```python
from build123d import *

# Parameters (mm, degrees)
ESQUISSE1_W             = 43
ESQUISSE1_H             = 43
BOSS_EXTRU_1_DEPTH      = 40
ESQUISSE2_W             = 48
ESQUISSE2_H             = 48
BOSS_EXTRU_2_DEPTH      = 1.5
ENL_V_MAT_EXTRU_3_REACH = 50
ESQUISSE5_W             = 8
ESQUISSE5_H             = 5
ENL_V_MAT_EXTRU_4_REACH = 43.5
ESQUISSE6_W             = 54.781223227
ESQUISSE6_H             = 3.078773465


with BuildPart() as part:
    # Esquisse1 → Boss.-Extru.1 (new body)
    with BuildSketch(Plane.XY):
        Polygon((-2.5, 43), (-2.5, -2.5), (0, -2.5), (45.5, -2.5), (45.5, 43), (45.5, 45.5), (-2.5, 45.5), align=None)
        with Locations((21.5, 21.5)):
            Rectangle(ESQUISSE1_W, ESQUISSE1_H, mode=Mode.SUBTRACT)
    extrude(amount=BOSS_EXTRU_1_DEPTH)

    # Esquisse2 → Boss.-Extru.2 (add)
    with BuildSketch(Plane.XY):
        with Locations((21.5, 21.5)):
            Rectangle(ESQUISSE2_W, ESQUISSE2_H)
    extrude(amount=-BOSS_EXTRU_2_DEPTH)

    # Esquisse5 → Enlèv. mat.-Extru.3 (cut, up to next)
    with BuildSketch(Plane(origin=(0, 45.5, 0), x_dir=(1, 0, 0), z_dir=(0, 1, 0)), mode=Mode.PRIVATE) as enl_v_mat_extru_3_sk1:
        with Locations((21.5, -6.3)):
            Rectangle(ESQUISSE5_W, ESQUISSE5_H)
    enl_v_mat_extru_3_tool1 = extrude(enl_v_mat_extru_3_sk1.sketch, amount=-ENL_V_MAT_EXTRU_3_REACH, mode=Mode.PRIVATE) & part.part
    add(enl_v_mat_extru_3_tool1.solids().sort_by_distance((21.5, 45.5, 6.3))[0], mode=Mode.SUBTRACT)

    # Esquisse6 → Enlèv. mat.-Extru.4 (cut, up to next)
    with BuildSketch(Plane.XY.offset(40), mode=Mode.PRIVATE) as enl_v_mat_extru_4_sk1:
        with Locations((23.162986277, -1.539386733)):
            Rectangle(ESQUISSE6_W, ESQUISSE6_H)
    enl_v_mat_extru_4_tool1 = extrude(enl_v_mat_extru_4_sk1.sketch, amount=-ENL_V_MAT_EXTRU_4_REACH, mode=Mode.PRIVATE) & part.part
    add(enl_v_mat_extru_4_tool1.solids().sort_by_distance((23.162986, -1.539387, 40))[0], mode=Mode.SUBTRACT)


solid = part.part
```
Verification items for the finished model (mm, model axes). A direction names the side the tool comes from. Give positions to 0.01 mm unless a question says otherwise; leave off trailing zeros. Loops run counter-clockwise (first coordinate to the right, second up) from the corner with the lowest first, then second, coordinate; pieces in that order, holes last. Notation, with made-up numbers: M 26,59.25 L 50,59.25 A25 ccw 50,86.25 Z; hole C 29,34.25 d9. An arc over 180 degrees is marked long. One line per question, with ' | ' between items.
Item 1: Depth check by flat-ended pin: P1, Ø20, axis at x = 15.5, z = 20.5, coming from the -Y side; P2, Ø13, axis at x = 22.5, y = 18.5, coming from the +Z side. Enter the tip coordinate at first touch or a pass-through.
Completed:
P1: stops at y = 43 | P2: stops at z = 0
Item 2: Tool access check on faces 1 (the face through (17.5, 44, 6)), 2 (the face through (45.5, 22, 20)), 3 (the face through (0, 21, 20)). Record the directions out of +Z, -Z, +X, -X, +Y, -Y that give a thin tool (end or side, any length) a straight path to the whole face; none if there is none.
Completed:
face 1: +Y, -Y | face 2: +Z, -Z, +X, +Y, -Y | face 3: +Z, -Y
Item 3: Thickness scan on line 1 (X direction, y = 29, z = 8); line 2 (Z direction, x = 18, y = 13); line 3 (Y direction, x = 6, z = 20). Record the ranges inside material, lowest first. Write a range as [from, to].
Completed:
line 1: x = [-2.5, 0], [43, 45.5] | line 2: z = [-1.5, 0] | line 3: y = [43, 45.5]
Item 4: Section check C-C, the plane y = 20.5. Record the cut outline in (x, z), plus the area to 3 significant figures.
Completed:
outline: M -2.5,-1.5 L 45.5,-1.5 L 45.5,40 L 43,40 L 43,0 L 0,0 L 0,40 L -2.5,40 Z | area: 272 mm^2
Item 5: Section check B-B, the plane x = 22.5. Record the cut outline in (y, z).
Completed:
outline: M 0,-1.5 L 45.5,-1.5 L 45.5,3.8 L 43,3.8 L 43,0 L 0,0 Z; M 43,8.8 L 45.5,8.8 L 45.5,40 L 43,40 Z
Item 6: Section check A-A, the plane z = 8. Record the cut outline in (x, y).
Completed:
outline: M -2.5,0 L 0,0 L 0,43 L 17.5,43 L 17.5,45.5 L -2.5,45.5 Z; M 25.5,43 L 43,43 L 43,0 L 45.5,0 L 45.5,45.5 L 25.5,45.5 Z
Item 7: Draft check along Z on faces 4 (the face through (21, 22, 0)), 5 (the face through (-2.5, 22, 20)), 6 (the face through (21, 44, 8.8)). Enter one of: +Z half, -Z half, draft (parallel to the pull), parting line (faces both ways), or undercut.
Completed:
face 4: +Z half | face 5: draft | face 6: undercut
Item 8: Section check D-D, the plane z = 22. Record the cut outline in (x, y), plus the area to 3 significant figures.
Completed:
outline: M -2.5,0 L 0,0 L 0,43 L 43,43 L 43,0 L 45.5,0 L 45.5,45.5 L -2.5,45.5 Z | area: 335 mm^2
